```python
from build123d import *

# Parameters (mm, degrees)
SKETCH1_R           = 55
SKETCH1_R_2         = 5
SKETCH1_R_3         = 1.75
BOSS_EXTRUDE1_DEPTH = 3


with BuildPart() as part:
    # Sketch1 → Boss-Extrude1 (new body)
    with BuildSketch(Plane(origin=(0, 0, 0), x_dir=(1, 0, 0), z_dir=(0, 1, 0))):
        with Locations(Location((0, 0, 0), (0, 0, 270))):
            Circle(SKETCH1_R)
        with Locations(Location((0, 0, 0), (0, 0, 270))):
            Circle(SKETCH1_R_2, mode=Mode.SUBTRACT)
        with Locations(Location((8.5, 0, 0), (0, 0, 270))):
            Circle(SKETCH1_R_3, mode=Mode.SUBTRACT)
        with Locations(Location((-8.5, 0, 0), (0, 0, 90))):
            Circle(SKETCH1_R_3, mode=Mode.SUBTRACT)
        with Locations(Location((-31.819805153, 31.819805153, 0), (0, 0, 270))):
            Circle(SKETCH1_R_3, mode=Mode.SUBTRACT)
        with Locations(Location((31.819805153, 31.819805153, 0), (0, 0, 270))):
            Circle(SKETCH1_R_3, mode=Mode.SUBTRACT)
        with Locations(Location((31.819805153, -31.819805153, 0), (0, 0, 270))):
            Circle(SKETCH1_R_3, mode=Mode.SUBTRACT)
        with Locations(Location((-31.819805153, -31.819805153, 0), (0, 0, 270))):
            Circle(SKETCH1_R_3, mode=Mode.SUBTRACT)
        with BuildLine():
            ThreePointArc((33.5, 0), (0, 33.5), (-33.5, 0))
            ThreePointArc((-33.5, 0), (-30, -3.5), (-26.5, 0))
            ThreePointArc((-26.5, 0), (0, 26.5), (26.5, 0))
            ThreePointArc((26.5, 0), (30, -3.5), (33.5, 0))
        make_face(mode=Mode.SUBTRACT)
    extrude(amount=BOSS_EXTRUDE1_DEPTH)


solid = part.part
```
Model file for the job. Use its own axes, mm. A direction names the side the tool comes from. Coordinates: 2 decimals unless noted, no trailing zeros. Loops run counter-clockwise (first coordinate to the right, second up) from the corner with the lowest first, then second, coordinate; pieces in that order, holes last. Notation, with made-up numbers: (27, -28.5) - (38, -28.5) arc R10 cw to (38, -11.5) - close; hole circle Ø7 at (7, 74). An arc over 180 degrees is marked (long way). Write item = value, one per line. Start each with the question number.
Item 1: Saw through at B-B, the plane z = -3. List the corners of the cut face in (x, y).
Item 2: Saw through at C-C, the plane y = 1.55. State how many separate pieces and enclosed holes the cut face has, then the cut area to 3 significant figures.
Item 3: Saw through at A-A, the plane x = 0. List the corners of the cut face in (y, z).
Item 4: Pull direction X, two halves, no side cores. Call faces 3 (the face through (-30.64, 1.48, 30.53)), 4 (the face through (-48.794, 1.479, 25.379)), 5 (the face through (1, 0, 11)): +X half, -X half, draft (parallel to the pull), parting line (faces both ways), or undercut.
Item 5: Wall check: probe 1 along X at (y, z) = (1.1, -24.5); probe 2 along X at (y, z) = (1.2, 30.5); probe 3 along Z at (x, y) = (-9, 2.45). Give the ranges that are in metal, low to high. Write a range as [from, to].
Item 6: Drop flat-ended pins along their axis: pin 1 Ø6 at (x, z) = (35, -24) entering from -Y; pin 2 Ø3 at (x, z) = (8.5, 0) entering from +Y. Give the stop position or say it passes through.
Item 7: Saw through at D-D, the plane z = 23. List the corners of the cut face in (x, y), then the cut area to 3 significant figures.
Item 8: 3-axis set-ups, long thin cutter, end or side, ignore diameter. For faces 1 (the face through (1, 3, 11)), 2 (the face through (29.9, 1.5, 3.5)): which of +Z, -Z, +X, -X, +Y, -Y reach the whole face in a straight line?
Answers:
q1.outline = (-54.92, 0) - (-33.37, 0) - (-33.37, 3) - (-54.92, 3) - close; (-26.33, 0) - (-4, 0) - (-4, 3) - (-26.33, 3) - close; (4, 0) - (26.33, 0) - (26.33, 3) - (4, 3) - close; (33.37, 0) - (54.92, 0) - (54.92, 3) - (33.37, 3) - close
q2.separate_pieces = 1
q2.enclosed_holes = 8
q2.area = 8,670 mm2
q3.outline = (0, -55) - (3, -55) - (3, -33.5) - (0, -33.5) - close; (0, -26.5) - (3, -26.5) - (3, -5) - (0, -5) - close; (0, 5) - (3, 5) - (3, 55) - (0, 55) - close
q4.face_3 = undercut
q4.face_4 = parting line
q4.face_5 = draft
q5.probe_1 = [-49.24, -22.85], [-10.1, 10.1], [22.85, 49.24]
q5.probe_2 = [-45.77, -32.97], [-30.67, 30.67], [32.97, 45.77]
q5.probe_3 = [-54.26, -32.27], [-24.92, -1.68], [1.68, 54.26]
q6.pin_1 = 0
q6.pin_2 = through
q7.outline = (-49.96, 0) - (49.96, 0) - (49.96, 3) - (-49.96, 3) - close
q7.area = 300 mm2
q8.face_1 = +Z, -Z, +X, -X, +Y
q8.face_2 = +Y, -Y
